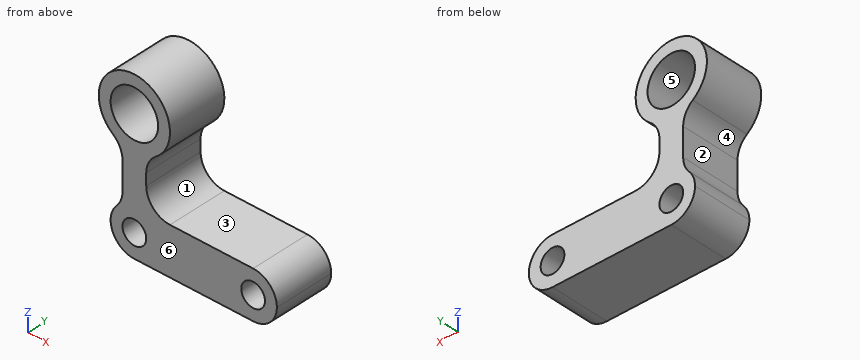
```python
from build123d import *

# Parameters (mm, degrees)
F0_R     = 5
F0_R_2   = 10
F1_DEPTH = 25


with BuildPart() as f1:
    # F0 (on Front) → F1 (new body)
    with BuildSketch(Plane.XZ):
        with BuildLine():
            ThreePointArc((-45.414113, -18.021473), (-42.48518, -25.092541), (-35.414113, -28.021473))
            Line((-35.414113, -28.021473), (14.585887, -28.021473))
            ThreePointArc((14.585887, -28.021473), (21.656955, -25.092541), (24.585887, -18.021473))
            ThreePointArc((24.585887, -18.021473), (21.656955, -10.950406), (14.585887, -8.021473))
            Line((14.585887, -8.021473), (-11.111964, -8.021473))
            Line((-11.111964, -8.021473), (-20.414113, -8.021473))
            ThreePointArc((-20.414113, -8.021473), (-27.48518, -5.092541), (-30.414113, 1.978527))
            Line((-30.414113, 1.978527), (-30.414113, 6.978527))
            ThreePointArc((-30.414113, 6.978527), (-29.358384, 11.450663), (-26.414113, 14.978527))
            ThreePointArc((-26.414113, 14.978527), (-35.414113, 41.978527), (-44.414113, 14.978527))
            ThreePointArc((-44.414113, 14.978527), (-41.469841, 11.450663), (-40.414113, 6.978527))
            Line((-40.414113, 6.978527), (-40.414113, -4.792717))
            ThreePointArc((-40.414113, -4.792717), (-41.059969, -8.328251), (-42.914113, -11.407095))
            ThreePointArc((-42.914113, -11.407095), (-44.768256, -14.48594), (-45.414113, -18.021473))
        make_face()
        with Locations((-35.414113, -18.021473)):
            Circle(F0_R, mode=Mode.SUBTRACT)
        with Locations((14.585887, -18.021473)):
            Circle(F0_R, mode=Mode.SUBTRACT)
        with Locations((-35.414113, 26.978527)):
            Circle(F0_R_2, mode=Mode.SUBTRACT)
    extrude(amount=F1_DEPTH)


solid = f1.part
```
Check sheet for the modelled part. Datum: model origin and axes. Units: mm. Face numbers are marked on the shaded views. A direction names the side the tool comes from. Coordinates: 2 decimals unless noted, no trailing zeros. Write each loop counter-clockwise with the first axis right and the second up, starting at its lowest first coordinate (ties: lowest second). Pieces come first, ordered by that corner, then holes. Notation, with made-up numbers: M 63,18.5 L 111,18.5 A30 ccw 111,55.5 Z; hole C -3.5,12.5 d6. An arc over 180 degrees is marked long. Write item = value, one per line. Start each with the question number.
1. Go/stop test with flat-tipped pins: pin 1 (9.5 mm diameter, centred on y = -9, z = 4, fed in from -X); pin 2 (2.5 mm diameter, centred on y = -11, z = 3.5, fed in from +X); pin 3 (12.5 mm diameter, centred on x = -4.5, y = -16.5, fed in from +Z); pin 4 (6 mm diameter, centred on x = -34.5, y = -16.5, fed in from +Z). Record where each tip stops, or that it passes through.
2. Sectioned sample at B-B (x = -24.5). Record the cut outline in (y, z).
3. Sectioned sample at D-D (y = -18). Record the cut outline in (x, z).
4. Tool access check on the marked faces 1, 2 and 3. Record the directions out of +Z, -Z, +X, -X, +Y, -Y that give a thin tool (end or side, any length) a straight path to the whole face; none if there is none.
5. Mould release check, pull along X, two halves, no side actions. Record for the marked faces 4, 5 and 6: pulls with the +X half, pulls with the -X half, needs draft (parallel to the pull), parting line crosses it, or undercut.
6. Thickness scan on probe 1 along Z at (x, y) = (-44.5, -11.75); probe 2 along X at (y, z) = (-1.75, 27); probe 3 along Z at (x, y) = (-29, -10.5). Record the ranges inside material, lowest first.
7. Sectioned sample at C-C (z = -15). Record the cut outline in (x, y).
8. Sectioned sample at A-A (z = 28). Record the cut outline in (x, y), then the cut area to 3 significant figures.
The answers:
q1.pin_1 = -40.57
q1.pin_2 = -30.41
q1.pin_3 = -8.02
q1.pin_4 = 41.98
q2.outline = M -25,-28.02 L 0,-28.02 L 0,-7.15 L -25,-7.15 Z; M -25,16.69 L 0,16.69 L 0,37.27 L -25,37.27 Z
q3.outline = M -45.41,-18.02 A10 ccw -35.41,-28.02 L 14.59,-28.02 A10 ccw 24.59,-18.02 A10 ccw 14.59,-8.02 L -20.41,-8.02 A10 cw -30.41,1.98 L -30.41,6.98 A10 cw -26.41,14.98 A15 ccw long -44.41,14.98 A10 cw -40.41,6.98 L -40.41,-4.79 A10 cw -42.91,-11.41 A10 ccw Z; hole C -35.41,26.98 d20; hole C -35.41,-18.02 d10; hole C 14.59,-18.02 d10
q4.face_1 = +X, +Y, -Y
q4.face_2 = -X, +Y, -Y
q4.face_3 = +Z, +X, +Y, -Y
q5.face_4 = pulls with the -X half
q5.face_5 = undercut
q5.face_6 = needs draft
q6.probe_1 = -22.2 to -13.84, 15.04 to 22.8, 31.16 to 38.91
q6.probe_2 = -50.41 to -45.41, -25.41 to -20.41
q6.probe_3 = -28.02 to -3.15, 12.11 to 19.31, 34.65 to 40.54
q7.outline = M -44.95,-25 L -39.4,-25 L -39.4,0 L -44.95,0 Z; M -31.43,-25 L 10.6,-25 L 10.6,0 L -31.43,0 Z; M 18.57,-25 L 24.12,-25 L 24.12,0 L 18.57,0 Z
q8.outline = M -50.38,-25 L -45.36,-25 L -45.36,0 L -50.38,0 Z; M -25.47,-25 L -20.45,-25 L -20.45,0 L -25.47,0 Z
q8.area = 251 mm²
